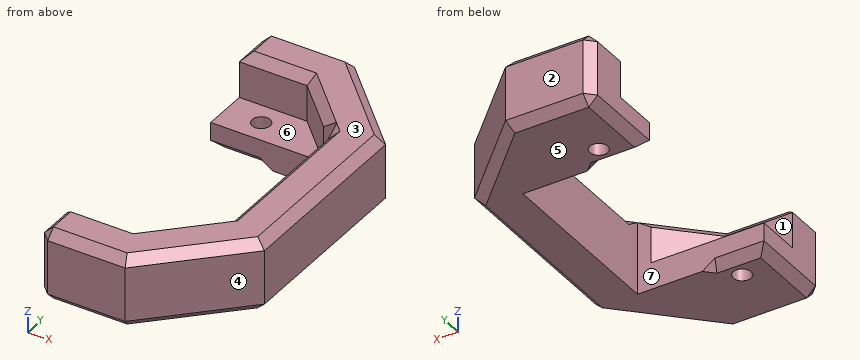
from build123d import *

# Parameters (mm, degrees)
EXTRUDE_1_DEPTH          = 3
EXTRUDE_2_DEPTH          = 5
SKETCH_4_R               = 1
CUT_EXTRUDE_1_DEPTH      = 8
CHAMFER_1_SIZE           = 1
CUT_EXTRUDE_3_DEPTH      = 26.690465157
CUT_EXTRUDE_3_DEPTH_BACK = 26.690465157


with BuildPart() as part:
    # 草图1 → 凸台-拉伸1 (new body)
    with BuildSketch(Plane.XY):
        Polygon((-5, -6.428932188), (-8.571067812, -10), (-14, -10), (-14, -15), (-6.5, -15), (0, -8.5), (0, 0), (0, 8.5), (-6.5, 15), (-14, 15), (-14, 10), (-8.571067812, 10), (-5, 6.428932188), (-5, 0), align=None)
        Polygon((-4.428932188, -20), (-14, -20), (-14, -15), (-6.5, -15), (0, -8.5), (0, 0), (0, 8.5), (-6.5, 15), (-14, 15), (-14, 20), (-4.428932188, 20), (5, 10.571067812), (5, 0), (5, -10.571067812), align=None)
    extrude(amount=EXTRUDE_1_DEPTH)

    # 草图3 → 凸台-拉伸2 (add)
    with BuildSketch(Plane.XY.offset(3)):
        Polygon((-14, -20), (-14, -15), (-6.5, -15), (0, -8.5), (0, 0), (0, 8.5), (-6.5, 15), (-14, 15), (-14, 20), (-4.428932188, 20), (5, 10.571067812), (5, 0), (5, -10.571067812), (-4.428932188, -20), align=None)
    extrude(amount=EXTRUDE_2_DEPTH)

    # 草图4 → 切除-拉伸1 (cut)
    with BuildSketch(Plane.XY.offset(3)):
        with Locations((-10, 12.5)):
            Circle(SKETCH_4_R)
        with Locations((-10, -12.5)):
            Circle(SKETCH_4_R)
    extrude(amount=-CUT_EXTRUDE_1_DEPTH, mode=Mode.SUBTRACT)

    # 倒角1
    chamfer_1_edges = [part.edges().sort_by_distance(p)[0] for p in [
        (-11.285533906, -10, 0),
        (-6.785533906, -8.214466094, 0),
        (-5, 0, 0),
        (-6.785533906, 8.214466094, 0),
        (-11.285533906, 10, 0),
        (-14, 15, 0),
        (-9.214466094, 20, 0),
        (0.285533906, 15.285533906, 0),
        (5, 0, 0),
        (0.285533906, -15.285533906, 0),
        (-9.214466094, -20, 0),
        (-14, -15, 0),
        (-14, 20, 4),
        (-14, -20, 4),
        (-9.214466094, -20, 8),
        (0.285533906, -15.285533906, 8),
        (5, 0, 8),
        (0.285533906, 15.285533906, 8),
        (-9.214466094, 20, 8),
        (-14, 17.5, 8),
        (-10.25, 15, 8),
        (-3.25, 11.75, 8),
        (0, 0, 8),
        (-3.25, -11.75, 8),
        (-10.25, -15, 8),
        (-14, -17.5, 8),
    ]]
    chamfer(chamfer_1_edges, length=CHAMFER_1_SIZE)

    # 草图6 → 切除-拉伸3 (cut, two sides: drawn at the far end of the back side and taken through both)
    with BuildSketch(Plane(origin=(0, 0, 0), x_dir=(-1, 0, 0), z_dir=(0, 0, -1)).offset(-CUT_EXTRUDE_3_DEPTH_BACK)):
        Polygon((84.424659409, 10), (8.571067812, 10), (0, 10), (0, -10), (8.571067812, -10), (84.424659409, -10), (236.131842603, -10), (236.131842603, 10), align=None)
    extrude(amount=CUT_EXTRUDE_3_DEPTH + CUT_EXTRUDE_3_DEPTH_BACK, mode=Mode.SUBTRACT)


solid = part.part
Here's how the part is built. I have some questions about the finished solid (model axes, mm). Face numbers are marked on the shaded views. A direction names the side the tool comes from. Coordinates: 2 decimals unless noted, no trailing zeros. Loops run counter-clockwise (first coordinate to the right, second up) from the corner with the lowest first, then second, coordinate; pieces in that order, holes last. Notation, with made-up numbers: (23, -27) -> (44, -27) arc R24 ccw to (44, 9) -> close; hole circle Ø7 at (41.5, 17). An arc over 180 degrees is marked (long way). Use one line per item in the form item = value. Start each with the question number.
(1) On a 3-axis mill with a long thin cutter (end or side, diameter ignored), from which of +Z, -Z, +X, -X, +Y, -Y can I reach the whole of each face in a straight line? I mean the marked faces 5, 6 and 7. Say none if no direction works.
(2) If we section it at B-B (z = 4.75): Please give me the cut outline in (x, y), then the cut area to 3 significant figures.
(3) Will these pins go through, and if not, where does the flat tip stop? pin 1 (1.5 mm diameter, centred on x = -6, y = -11.5, fed in from +Z); pin 2 (4 mm diameter, centred on y = 1.5, z = 3, fed in from -X); pin 3 (1.8 mm diameter, centred on x = -10, y = -12.5, fed in from +Z); pin 4 (2 mm diameter, centred on x = -5.5, y = -13, fed in from +Z).
(4) If we section it at D-D (x = -3.5): Please give me the cut outline in (y, z).
(5) If we section it at A-A (y = 7): Please give me the cut outline in (x, z).
(6) Please list where these lines run through material, in increasing order: line 1 along Y through (x, z) = (-10, 1.45); line 2 along Y through (x, z) = (-10, 3.5); line 3 along Y through (x, z) = (-0.25, 5.25).
(7) If we section it at C-C (x = -10): Please give me the cut outline in (y, z), then the cut area to 3 significant figures.
(8) We'd pull the mould along Y, two halves only. Please class the marked faces 1, 2, 3 and 4: pulls with the +Y half, pulls with the -Y half, needs draft (parallel to the pull), parting line crosses it, or undercut.
Verdict:
q1.face_5 = -Z, +X, -X, +Y, -Y
q1.face_6 = +Z, -X
q1.face_7 = +Z, -Z, -X
q2.outline = (-14, -19) -> (-13, -20) -> (-4.43, -20) -> (5, -10.57) -> (5, 10.57) -> (-4.43, 20) -> (-13, 20) -> (-14, 19) -> (-14, 15) -> (-6.5, 15) -> (-1.5, 10) -> (0, 10) -> (0, -10) -> (-1.5, -10) -> (-6.5, -15) -> (-14, -15) -> close
q2.area = 290 mm²
q3.pin_1 = 3
q3.pin_2 = 0
q3.pin_3 = through
q3.pin_4 = 7.29
q4.outline = (-19.07, 1) -> (-17.66, 0) -> (-10, 0) -> (-10, 3) -> (-12, 3) -> (-12, 7) -> (-13.41, 8) -> (-17.66, 8) -> (-19.07, 7) -> close; (10, 0) -> (17.66, 0) -> (19.07, 1) -> (19.07, 7) -> (17.66, 8) -> (13.41, 8) -> (12, 7) -> (12, 3) -> (10, 3) -> close
q5.outline = (0, 0) -> (4, 0) -> (5, 1) -> (5, 7) -> (4, 8) -> (1, 8) -> (0, 7) -> close
q6.line_1 = -20 to -13.5, -11.5 to -10, 10 to 11.5, 13.5 to 20
q6.line_2 = -20 to -15, 15 to 20
q6.line_3 = -15.82 to -10, 10 to 15.82
q7.outline = (-20, 1) -> (-19, 0) -> (-13.5, 0) -> (-13.5, 3) -> (-15, 3) -> (-15, 7) -> (-16, 8) -> (-19, 8) -> (-20, 7) -> close; (-11.5, 0) -> (-11, 0) -> (-10, 1) -> (-10, 3) -> (-11.5, 3) -> close; (10, 1) -> (11, 0) -> (11.5, 0) -> (11.5, 3) -> (10, 3) -> close; (13.5, 0) -> (19, 0) -> (20, 1) -> (20, 7) -> (19, 8) -> (16, 8) -> (15, 7) -> (15, 3) -> (13.5, 3) -> close
q7.area = 94.0 mm²
q8.face_1 = undercut
q8.face_2 = pulls with the +Y half
q8.face_3 = needs draft
q8.face_4 = pulls with the -Y half
